Can you work these out from the model? Positions are in its coordinate system, mm. Face numbers are marked on the shaded views. A direction names the side the tool comes from. Give positions to 0.01 mm unless a question says otherwise; leave off trailing zeros. Write each loop counter-clockwise with the first axis right and the second up, starting at its lowest first coordinate (ties: lowest second). Pieces come first, ordered by that corner, then holes.
from build123d import *

# Parameters (mm, degrees)
SKETCH_1_W          = 181
SKETCH_1_H          = 30
EXTRUDE_1_DEPTH     = 2
SKETCH_2_W          = 181
SKETCH_2_H          = 2
EXTRUDE_2_DEPTH     = 10
SKETCH_3_W          = 181
SKETCH_3_H          = 32
EXTRUDE_3_DEPTH     = 2
CUT_EXTRUDE_1_DEPTH = 2
SKETCH_5_W          = 12
SKETCH_5_H          = 20.057389113
EXTRUDE_4_DEPTH     = 2
SKETCH_6_W          = 12
SKETCH_6_H          = 20.057389113
EXTRUDE_5_DEPTH     = 2
FILLET_1_R          = 1


with BuildPart() as part:
    # 草图1 → 凸台-拉伸1 (new body)
    with BuildSketch(Plane.XY):
        with Locations((90.5, 15)):
            Rectangle(SKETCH_1_W, SKETCH_1_H)
    extrude(amount=EXTRUDE_1_DEPTH)

    # 草图2 → 凸台-拉伸2 (add)
    with BuildSketch(Plane.XY):
        with Locations((90.5, -1)):
            Rectangle(SKETCH_2_W, SKETCH_2_H)
    extrude(amount=EXTRUDE_2_DEPTH)

    # 草图3 → 凸台-拉伸3 (add)
    with BuildSketch(Plane.XY.offset(10)):
        with Locations((90.5, 14)):
            Rectangle(SKETCH_3_W, SKETCH_3_H)
    extrude(amount=EXTRUDE_3_DEPTH)

    # 草图4 → 切除-拉伸1 (cut)
    with BuildSketch(Plane.XY.offset(12)):
        with BuildLine():
            Line((19.5, 6), (19.5, 10))
            Line((19.5, 10), (19.5, 14))
            ThreePointArc((19.5, 14), (18.5, 15), (17.5, 14))
            Line((17.5, 14), (17.5, 6))
            ThreePointArc((17.5, 6), (18.5, 5), (19.5, 6))
        make_face()
        with BuildLine():
            Line((21.5, 14), (21.5, 6))
            ThreePointArc((21.5, 6), (22.5, 5), (23.5, 6))
            Line((23.5, 6), (23.5, 14))
            ThreePointArc((23.5, 14), (22.5, 15), (21.5, 14))
        make_face()
        with BuildLine():
            Line((157.5, 14), (157.5, 6))
            ThreePointArc((157.5, 6), (158.5, 5), (159.5, 6))
            Line((159.5, 6), (159.5, 14))
            ThreePointArc((159.5, 14), (158.5, 15), (157.5, 14))
        make_face()
        with BuildLine():
            Line((91.5, 14), (91.5, 6))
            ThreePointArc((91.5, 6), (92.5, 5), (93.5, 6))
            Line((93.5, 6), (93.5, 14))
            ThreePointArc((93.5, 14), (92.5, 15), (91.5, 14))
        make_face()
        with BuildLine():
            Line((87.5, 14), (87.5, 6))
            ThreePointArc((87.5, 6), (88.5, 5), (89.5, 6))
            Line((89.5, 6), (89.5, 14))
            ThreePointArc((89.5, 14), (88.5, 15), (87.5, 14))
        make_face()
        with BuildLine():
            Line((163.5, 6), (163.5, 14))
            ThreePointArc((163.5, 14), (162.5, 15), (161.5, 14))
            Line((161.5, 14), (161.5, 6))
            ThreePointArc((161.5, 6), (162.5, 5), (163.5, 6))
        make_face()
    extrude(amount=-CUT_EXTRUDE_1_DEPTH, mode=Mode.SUBTRACT)

    # 草图5 → 凸台-拉伸4 (add)
    with BuildSketch(Plane(origin=(0, 0, 0), x_dir=(0, 0, -1), z_dir=(1, 0, 0))):
        with Locations((-6, 8.028694557)):
            Rectangle(SKETCH_5_W, SKETCH_5_H)
    extrude(amount=-EXTRUDE_4_DEPTH)

    # 草图6 → 凸台-拉伸5 (add)
    with BuildSketch(Plane(origin=(181, 0, 0), x_dir=(0, 0, -1), z_dir=(1, 0, 0))):
        with Locations((-6, 8.028694557)):
            Rectangle(SKETCH_6_W, SKETCH_6_H)
    extrude(amount=EXTRUDE_5_DEPTH)

    # 圆角1
    fillet_1_edges = [part.edges().sort_by_distance(p)[0] for p in [
        (-2, 18.057389113, 6),
        (183, 18.057389113, 6),
        (181, 30, 11),
        (0, 30, 11),
        (0, 30, 1),
        (181, 30, 1),
    ]]
    fillet(fillet_1_edges, radius=FILLET_1_R)


solid = part.part
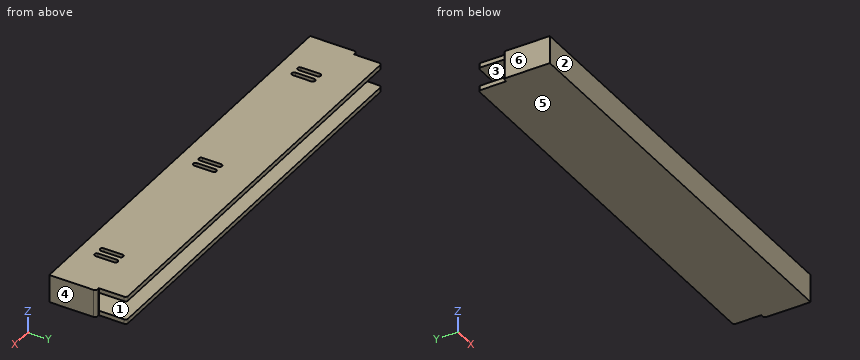
(1) If we mould it in two halves opening along X, with no side actions, what happens to the marked faces 3, 4, 5 and 6? For each: +X half, -X half, draft (parallel to the pull), parting line (faces both ways), or undercut.
Returned:
face 3: undercut
face 4: +X half
face 5: draft
face 6: -X half
(2) Imagine slicing it at C-C, the plane z = 6. Write out the boundary of the cut face in (x, y), plus the area to 3 significant figures.
Returned:
outline: (-2, -2) - (183, -2) - (183, 17.06) arc R1 ccw to (182, 18.06) - (181, 18.06) - (181, 0) - (0, 0) - (0, 18.06) - (-1, 18.06) arc R1 ccw to (-2, 17.06) - close
area: 442 mm2
(3) Imagine slicing it at B-B, the plane y = 9. Give the number of separate pieces and of enclosed holes in the cut face, plus the area to 3 significant figures.
Returned:
separate pieces: 6
enclosed holes: 0
area: 748 mm2
(4) If I drill on L1, parallel to X at y = 10, z = 5.5; L2, parallel to Z at x = 93.5, y = 24; L3, parallel to Y at x = 24, z = 6, over which ranges is the centre line in solid material (lowest first)?
Returned:
L1: x = -2 to 0, 181 to 183
L2: z = 0 to 2, 10 to 12
L3: y = -2 to 0
(5) Imagine slicing it at A-A, the plane x = 63. Write out the boundary of the cut face in (y, z), plus the area to 3 significant figures.
Returned:
outline: (-2, 0) - (30, 0) - (30, 2) - (0, 2) - (0, 10) - (30, 10) - (30, 12) - (-2, 12) - close
area: 144 mm2
(6) For the marked faces 1 and 2, which set-ups out of +Z, -Z, +X, -X, +Y, -Y let a thin tool reach every point of the face, with its end or its side?
Returned:
face 1: +Y
face 2: +Z, -Z, +X, -X, -Y
(7) Will these pins go through, and if not, where does the flat tip stop? P1, Ø1, axis at y = 26, z = 1, coming from the +X side; P2, Ø0.8, axis at x = 181.5, z = 8, coming from the +Y side; P3, Ø3, axis at x = 119.5, y = 13.5, coming from the -Z side; P4, Ø4, axis at x = 97, z = 5, coming from the +Y side.
Returned:
P1: stops at x = 181
P2: stops at y = 18.06
P3: stops at z = 0
P4: stops at y = 0
